from build123d import *

# Parameters (mm, degrees)
SKETCH1_W           = 80
SKETCH1_H           = 100
SKETCH1_R           = 21.5
SKETCH1_R_2         = 14
SKETCH1_R_3         = 2
BOSS_EXTRUDE1_DEPTH = 5
SKETCH3_W           = 80
SKETCH3_H           = 55.127756358
CUT_EXTRUDE1_DEPTH  = 6


with BuildPart() as part:
    # Sketch1 → Boss-Extrude1 (new body)
    with BuildSketch(Plane(origin=(0, 0, 0), x_dir=(0, 0, -1), z_dir=(1, 0, 0))):
        Rectangle(SKETCH1_W, SKETCH1_H)
        with BuildLine():
            ThreePointArc((24, -39), (20, -35), (16, -39))
            Line((16, -39), (16, -41))
            ThreePointArc((16, -41), (20, -45), (24, -41))
            Line((24, -41), (24, -39))
        make_face(mode=Mode.SUBTRACT)
        with BuildLine():
            ThreePointArc((-24, 39), (-20, 35), (-16, 39))
            Line((-16, 39), (-16, 41))
            ThreePointArc((-16, 41), (-20, 45), (-24, 41))
            Line((-24, 41), (-24, 39))
        make_face(mode=Mode.SUBTRACT)
        with BuildLine():
            Line((24, 41), (24, 39))
            ThreePointArc((24, 39), (20, 35), (16, 39))
            Line((16, 39), (16, 41))
            ThreePointArc((16, 41), (20, 45), (24, 41))
        make_face(mode=Mode.SUBTRACT)
        with BuildLine():
            Line((-24, -41), (-24, -39))
            ThreePointArc((-24, -39), (-20, -35), (-16, -39))
            Line((-16, -39), (-16, -41))
            ThreePointArc((-16, -41), (-20, -45), (-24, -41))
        make_face(mode=Mode.SUBTRACT)
        with BuildLine():
            Line((40, -50), (-40, -50))
            Line((-40, -50), (-18.452584301, -86.034134882))
            ThreePointArc((-18.452584301, -86.034134882), (-5.72361064, -54.275852702), (21.5, -75))
            ThreePointArc((21.5, -75), (20.724147298, -80.72361064), (18.452584301, -86.034134882))
            Line((18.452584301, -86.034134882), (40, -50))
        make_face()
        with Locations((0, -75)):
            Circle(SKETCH1_R)
        with Locations((0, -75)):
            Circle(SKETCH1_R_2, mode=Mode.SUBTRACT)
        with Locations((17.5, -75)):
            Circle(SKETCH1_R_3, mode=Mode.SUBTRACT)
        with Locations((0, -92.5)):
            Circle(SKETCH1_R_3, mode=Mode.SUBTRACT)
        with Locations((-17.5, -75)):
            Circle(SKETCH1_R_3, mode=Mode.SUBTRACT)
        with Locations((0, -57.5)):
            Circle(SKETCH1_R_3, mode=Mode.SUBTRACT)
    extrude(amount=BOSS_EXTRUDE1_DEPTH)

    # Sketch3 → Cut-Extrude1 (cut, through all)
    with BuildSketch(Plane(origin=(5, 0, 0), x_dir=(0, 0, -1), z_dir=(1, 0, 0))):
        with Locations((0, -77.563878179)):
            Rectangle(SKETCH3_W, SKETCH3_H)
    extrude(amount=-CUT_EXTRUDE1_DEPTH, mode=Mode.SUBTRACT)


solid = part.part
The model under review builds one solid part; all positions refer to its coordinate system, in mm. A direction names the side the tool comes from. Give positions to 0.01 mm unless a question says otherwise; leave off trailing zeros. Order: outer loops, then holes, each group sorted by start corner. A loop starts at its lowest first (then second) coordinate and runs counter-clockwise, first axis right, second up. Notation, with made-up numbers: M 5,21 L 44,21 A16 ccw 44,26 Z; hole C 28,63.5 d10. An arc over 180 degrees is marked long. One line per question, with ' | ' between items. Start each with the question number.
1) For faces 4 (the face through (5, 1, 1)), 5 (the face through (2, -40, -16)), list the 3-axis set-ups (+Z, -Z, +X, -X, +Y, -Y) from which the entire face can be reached by the end or side of a thin tool; tool diameter is ignored.
2) Mouldability with a two-part tool opening along Y and no side actions: class faces 1 (the face through (2, 45, -20)), 2 (the face through (2, -1, 40)), 3 (the face through (3, -50, 1)) as pulls with the +Y half, pulls with the -Y half, needs draft (parallel to the pull), parting line crosses it, or undercut.
3) Wall thickness on L1, parallel to Y at x = 3.5, z = -21; L2, parallel to Y at x = 1.55, z = -22.5; L3, parallel to Z at x = 4.2, y = 43: over which ranges is each line inside the solid? List them lowest first. Write a range as from..to.
4) Consider section B-B, the plane x = 4.25. Give the boundary of the cut face in (y, z), then the cut area to 3 significant figures.
5) Consider section A-A, the plane z = 20. Give the boundary of the cut face in (x, y), then the cut area to 3 significant figures.
Found:
1) face 4: +Z, -Z, +X, +Y, -Y | face 5: +X, -X
2) face 1: undercut | face 2: needs draft | face 3: pulls with the -Y half
3) L1: y = -50..-44.87, -35.13..35.13, 44.87..50 | L2: y = -50..-44.12, -35.88..35.88, 44.12..50 | L3: z = -40..-23.46, -16.54..16.54, 23.46..40
4) outline: M -50,-40 L 50,-40 L 50,40 L -50,40 Z; hole M -41,-24 L -39,-24 A4 ccw -39,-16 L -41,-16 A4 ccw Z; hole M -41,16 L -39,16 A4 ccw -39,24 L -41,24 A4 ccw Z; hole M 39,-24 L 41,-24 A4 ccw 41,-16 L 39,-16 A4 ccw Z; hole M 39,16 L 41,16 A4 ccw 41,24 L 39,24 A4 ccw Z | area: 7,730 mm²
5) outline: M 0,-50 L 5,-50 L 5,-45 L 0,-45 Z; M 0,-35 L 5,-35 L 5,35 L 0,35 Z; M 0,45 L 5,45 L 5,50 L 0,50 Z | area: 400 mm²
